Verification items for the finished model (mm, model axes). Coordinates: 2 decimals unless noted, no trailing zeros. Write each loop counter-clockwise with the first axis right and the second up, starting at its lowest first coordinate (ties: lowest second). Pieces come first, ordered by that corner, then holes. Notation, with made-up numbers: (34, 30) -> (71, 30) arc R29 ccw to (71, 66) -> close; hole circle Ø2 at (76.25, -9). An arc over 180 degrees is marked (long way). Write item = value, one per line. Start each with the question number.
(1) Section check C-C (z = 18). Record the cut outline in (x, y).
(2) Mould release check, pull along Y, two halves, no side actions. Record for faces 1 (the face through (0, -3, 7)), 2 (the face through (3.131, 205.715, -4.292)): released by +Y, released by -Y, zero draft, split by the parting line, or undercut.
(3) Material ranges on probe 1 along Z at (x, y) = (3.5, -215.9); probe 2 along Y at (x, z) = (4.25, -12); probe 3 along Y at (x, z) = (3.25, -12.5), recorded low to high. Write a range as [from, to].
(4) Section check B-B (y = -88.9). Record the cut outline in (x, z).
(5) Section check A-A (x = 3.5). State how many separate pieces and enclosed holes the cut face has, plus the area to 3 significant figures.
(6) Gauge pin test, flat ends, axial feed: pin 1 Ø1.5 at (x, z) = (5, 25) entering from -Y; pin 2 Ø7.5 at (y, z) = (215.9, 0) entering from +X. Record the tip position at first contact, or that the pin passes through.
(7) Section check D-D (y = -136). Record the cut outline in (x, z), plus the area to 3 significant figures.
```python
from build123d import *

# Parameters (mm, degrees)
F0_W     = 114.3
F0_H     = 25.4
F0_R     = 2.54
F0_R_2   = 14.2875
F1_DEPTH = 6.35
F2_R     = 5.08


with BuildPart() as f1:
    # F0 (on Right) → F1 (new body)
    with BuildSketch(Plane.YZ):
        with Locations((-171.45, -12.7)):
            Rectangle(F0_W, F0_H)
        with Locations((-215.9, -12.7)):
            Circle(F0_R, mode=Mode.SUBTRACT)
        Polygon((228.6, 38.1), (-114.3, 38.1), (-114.3, 0), (-114.3, -25.4), (228.6, -25.4), (228.6, 0), align=None)
        with Locations((-88.9, 0)):
            Circle(F0_R_2, mode=Mode.SUBTRACT)
        with BuildLine():
            ThreePointArc((165.1, 0), (168.275, 3.175), (171.45, 0))
            ThreePointArc((171.45, 0), (168.275, -3.175), (165.1, 0))
        make_face(mode=Mode.SUBTRACT)
        with BuildLine():
            ThreePointArc((177.8, 0), (192.0875, 14.2875), (206.375, 0))
            ThreePointArc((206.375, 0), (192.0875, -14.2875), (177.8, 0))
        make_face(mode=Mode.SUBTRACT)
        with BuildLine():
            ThreePointArc((212.725, 0), (215.9, 3.175), (219.075, 0))
            ThreePointArc((219.075, 0), (215.9, -3.175), (212.725, 0))
        make_face(mode=Mode.SUBTRACT)
    extrude(amount=F1_DEPTH)

    # F2
    f2_edges = [f1.edges().sort_by_distance(p)[0] for p in [
        (3.175, -114.3, 0),
        (3.175, -114.3, 38.1),
        (3.175, -228.6, 0),
        (3.175, -228.6, -25.4),
        (3.175, 228.6, 38.1),
        (3.175, 228.6, -25.4),
    ]]
    fillet(f2_edges, radius=F2_R)


solid = f1.part
```
Response:
q1.outline = (0, -114.3) -> (6.35, -114.3) -> (6.35, 228.6) -> (0, 228.6) -> close
q2.face_1 = zero draft
q2.face_2 = undercut
q3.probe_1 = [-25.4, -15.24], [-10.16, 0]
q3.probe_2 = [-228.6, -218.34], [-213.46, -96.65], [-81.15, 184.33], [199.84, 228.6]
q3.probe_3 = [-228.6, -218.43], [-213.37, -95.82], [-81.98, 185.17], [199.01, 228.6]
q4.outline = (0, -25.4) -> (6.35, -25.4) -> (6.35, -14.29) -> (0, -14.29) -> close; (0, 14.29) -> (6.35, 14.29) -> (6.35, 38.1) -> (0, 38.1) -> close
q5.separate_pieces = 1
q5.enclosed_holes = 5
q5.area = 23,300 mm2
q6.pin_1 = -114.3
q6.pin_2 = 6.35
q7.outline = (0, -25.4) -> (6.35, -25.4) -> (6.35, 0) -> (0, 0) -> close
q7.area = 161 mm2
